from build123d import *

# Parameters (mm, degrees)
SKETCH1_W                   = 50.8
SKETCH1_H                   = 76.2
BOSS_EXTRUDE1_DEPTH         = 6.35
F_1_4_20_TAPPED_HOLE1_D     = 5.1054
F_1_4_20_TAPPED_HOLE1_DEPTH = 19.05
F_1_4_20_TAPPED_HOLE1_TIP   = 1.533816902
CUT_EXTRUDE1_REACH          = 14.7
SKETCH5_W                   = 25.4
SKETCH5_H                   = 0.635
F_1_4_20_TAPPED_HOLE2_D     = 5.1054
F_1_4_20_TAPPED_HOLE2_DEPTH = 19.05
F_1_4_20_TAPPED_HOLE2_TIP   = 1.533816902
CUT_EXTRUDE2_REACH          = 14.7
SKETCH8_R                   = 12.7
SKETCH9_W                   = 22.225
SKETCH9_H                   = 19.05
BOSS_EXTRUDE2_DEPTH         = 12.7
F_8_32_TAPPED_HOLE1_D       = 3.4544
SKETCH12_R                  = 4.7625
CUT_EXTRUDE3_DEPTH          = 26.4
F_8_32_TAPPED_HOLE2_D       = 3.4544


with BuildPart() as part:
    # Sketch1 → Boss-Extrude1 (new body, symmetric)
    with BuildSketch(Plane(origin=(0, 0, 0), x_dir=(0, 0, -1), z_dir=(1, 0, 0))):
        Rectangle(SKETCH1_W, SKETCH1_H)
    extrude(amount=BOSS_EXTRUDE1_DEPTH, both=True)

    # 1/4-20 Tapped Hole1
    with Locations(Plane(origin=(0, -38.1, 0), x_dir=(-1, 0, 0), z_dir=(0, -1, 0))):
        with Locations((0, -19.05), (0, 19.05)):
            Hole(F_1_4_20_TAPPED_HOLE1_D / 2, depth=F_1_4_20_TAPPED_HOLE1_DEPTH)
            with Locations((0, 0, -(F_1_4_20_TAPPED_HOLE1_DEPTH + F_1_4_20_TAPPED_HOLE1_TIP / 2))):  # 118° drill point
                Cone(0, F_1_4_20_TAPPED_HOLE1_D / 2, F_1_4_20_TAPPED_HOLE1_TIP, mode=Mode.SUBTRACT)

    # Sketch5 → Cut-Extrude1 (cut, up to next)
    with BuildSketch(Plane(origin=(6.35, 0, 0), x_dir=(0, 0, -1), z_dir=(1, 0, 0)), mode=Mode.PRIVATE) as cut_extrude1_sk1:
        with Locations((0, -37.7825)):
            Rectangle(SKETCH5_W, SKETCH5_H)
    cut_extrude1_tool1 = extrude(cut_extrude1_sk1.sketch, amount=-CUT_EXTRUDE1_REACH, mode=Mode.PRIVATE) & part.part
    add(cut_extrude1_tool1.solids().sort_by_distance((6.35, -37.7825, 0))[0], mode=Mode.SUBTRACT)

    # 1/4-20 Tapped Hole2
    with Locations(Plane(origin=(0, 38.1, 0), x_dir=(1, 0, 0), z_dir=(0, 1, 0))):
        with Locations((0, 19.05), (0, 0), (0, -19.05)):
            Hole(F_1_4_20_TAPPED_HOLE2_D / 2, depth=F_1_4_20_TAPPED_HOLE2_DEPTH)
            with Locations((0, 0, -(F_1_4_20_TAPPED_HOLE2_DEPTH + F_1_4_20_TAPPED_HOLE2_TIP / 2))):  # 118° drill point
                Cone(0, F_1_4_20_TAPPED_HOLE2_D / 2, F_1_4_20_TAPPED_HOLE2_TIP, mode=Mode.SUBTRACT)

    # Sketch8 → Cut-Extrude2 (cut, up to next)
    with BuildSketch(Plane(origin=(6.35, 0, 0), x_dir=(0, 0, -1), z_dir=(1, 0, 0)), mode=Mode.PRIVATE) as cut_extrude2_sk1:
        with Locations((0, -7.62)):
            Circle(SKETCH8_R)
    cut_extrude2_tool1 = extrude(cut_extrude2_sk1.sketch, amount=-CUT_EXTRUDE2_REACH, mode=Mode.PRIVATE) & part.part
    add(cut_extrude2_tool1.solids().sort_by_distance((6.35, -7.62, 0))[0], mode=Mode.SUBTRACT)

    # Sketch9 → Boss-Extrude2 (add)
    with BuildSketch(Plane.ZY.offset(6.35)):
        with Locations((-14.2875, 28.575)):
            Rectangle(SKETCH9_W, SKETCH9_H)
    extrude(amount=BOSS_EXTRUDE2_DEPTH)

    # #8-32 Tapped Hole1 (through all)
    with Locations(Plane.XY.offset(-3.175)):
        with Locations((-15.24, 30.48)):
            Hole(F_8_32_TAPPED_HOLE1_D / 2)

    # Sketch12 → Cut-Extrude3 (cut, through all)
    with BuildSketch(Plane(origin=(6.35, 0, 0), x_dir=(0, 0, -1), z_dir=(1, 0, 0))):
        with Locations((0, 15.24)):
            Circle(SKETCH12_R)
    extrude(amount=-CUT_EXTRUDE3_DEPTH, mode=Mode.SUBTRACT)

    # #8-32 Tapped Hole2 (through all)
    with Locations(Plane.XY.offset(25.4)):
        with Locations((0, -7.62)):
            Hole(F_8_32_TAPPED_HOLE2_D / 2)


solid = part.part
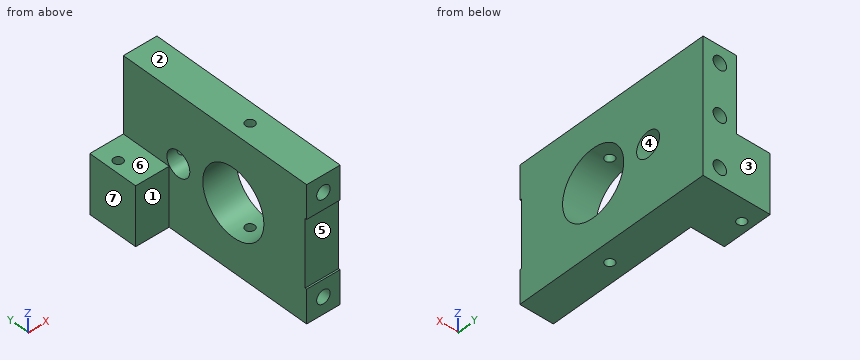
Check sheet for the modelled part. Datum: model origin and axes. Units: mm. Face numbers are marked on the shaded views. A direction names the side the tool comes from. Coordinates: 2 decimals unless noted, no trailing zeros. Write each loop counter-clockwise with the first axis right and the second up, starting at its lowest first coordinate (ties: lowest second). Pieces come first, ordered by that corner, then holes. Notation, with made-up numbers: M -26.5,6 L 31.5,6 A22 ccw 31.5,40 Z; hole C 75.5,69.5 d11. An arc over 180 degrees is marked long. Answer as CSV lines item,"result".
Q1. Set-up check for the marked faces 5, 6 and 7: record each of +Z, -Z, +X, -X, +Y, -Y from which the full face is reachable in a straight line by a thin tool's end or side.
Check result:
face 5,"+X, -X, -Y"
face 6,"+Z, -X, +Y, -Y"
face 7,"+Z, -Z, -X, +Y, -Y"
Q2. Cross-section at B-B (z = 0). Count the separate pieces of the cut face and the enclosed holes in it, then the cut area to 3 significant figures.
Check result:
separate pieces,"4"
enclosed holes,"0"
area,"424 mm^2"
Q3. Cross-section at D-D (y = -7.62). Record the boundary of the cut face in (x, z), then the cut area to 3 significant figures.
Check result:
outline,"M -6.35,-25.4 L -1.73,-25.4 L -1.73,-12.7 L -6.35,-12.7 Z; M -6.35,12.7 L -1.73,12.7 L -1.73,25.4 L -6.35,25.4 Z; M 1.73,-25.4 L 6.35,-25.4 L 6.35,-12.7 L 1.73,-12.7 Z; M 1.73,12.7 L 6.35,12.7 L 6.35,25.4 L 1.73,25.4 Z"
area,"235 mm^2"
Q4. Material ranges on probe 1 along Z at (x, y) = (0, 28.5); probe 2 along Z at (x, y) = (0, -32.25); probe 3 along X at (y, z) = (33, 19), recorded low to high. Write a range as from..to.
Check result:
probe 1,"-25.4..-21.6, -16.5..-2.55, 2.55..16.5, 21.6..25.4"
probe 2,"-25.4..-21.6, -16.5..16.5, 21.6..25.4"
probe 3,"-6.35..-2.55, 2.55..6.35"
Q5. Mould release check, pull along Y, two halves, no side actions. Record for the marked faces 1, 2, 3 and 4: released by +Y, released by -Y, zero draft, split by the parting line, or undercut.
Check result:
face 1,"released by -Y"
face 2,"zero draft"
face 3,"released by +Y"
face 4,"undercut"
Q6. Cross-section at A-A (y = 30.48). Record the boundary of the cut face in (x, z) (3 decimals), then the cut area to 3 significant figures.
Check result:
outline,"M -19.05,-25.4 L -16.967,-25.4 L -16.967,-3.175 L -19.05,-3.175 Z; M -13.513,-25.4 L 6.35,-25.4 L 6.35,25.4 L -6.35,25.4 L -6.35,-3.175 L -13.513,-3.175 Z; hole C 0,-19.05 d5.105; hole C 0,0 d5.105; hole C 0,19.05 d5.105"
area,"789 mm^2"
Q7. Cross-section at C-C (x = -15.5). Record the boundary of the cut face in (y, z) (3 decimals).
Check result:
outline,"M 19.05,-25.4 L 28.772,-25.4 L 28.772,-3.175 L 19.05,-3.175 Z; M 32.188,-25.4 L 38.1,-25.4 L 38.1,-3.175 L 32.188,-3.175 Z"
Q8. Go/stop test with flat-tipped pins: pin 1 (4 mm diameter, centred on x = 0.5, z = -2.5, fed in from -Y) (3 decimals); pin 2 (15 mm diameter, centred on y = 10.5, z = -2, fed in from -X); pin 3 (6.5 mm diameter, centred on x = -11, y = 28, fed in from +Z) (3 decimals); pin 4 (2 mm diameter, centred on x = -15.24, y = 30.48, fed in from -Z). Record where each tip stops, or that it passes through.
Check result:
pin 1,"y = -37.465"
pin 2,"x = -6.35"
pin 3,"z = -3.175"
pin 4,"through"
